```python
from build123d import *

# Parameters (mm, degrees)
SKETCH_1_R               = 5
SKETCH_1_W               = 40
SKETCH_1_H               = 6
EXTRUDE_1_DEPTH          = 2
CUT_EXTRUDE_2_DEPTH      = 46.44227107
CUT_EXTRUDE_2_DEPTH_BACK = 46.44227107
SKETCH_1_3_R             = 2
FILLET_1_R               = 3


with BuildPart() as part:
    # 草图1 → 凸台-拉伸1 (new body)
    with BuildSketch(Plane(origin=(0, 0, 0), x_dir=(0, 0, -1), z_dir=(1, 0, 0))):
        Circle(SKETCH_1_R)
        with Locations((40, -1)):
            Circle(SKETCH_1_R)
        with Locations((20, 0)):
            Rectangle(SKETCH_1_W, SKETCH_1_H)
    extrude(amount=EXTRUDE_1_DEPTH)

    # 草图1<3> → 切除-拉伸2 (cut, two sides: drawn at the far end of the back side and taken through both)
    with BuildSketch(Plane(origin=(0, 0, 0), x_dir=(0, 0, -1), z_dir=(1, 0, 0)).offset(-CUT_EXTRUDE_2_DEPTH_BACK)):
        Circle(SKETCH_1_3_R)
        with Locations((40, -1)):
            Circle(SKETCH_1_3_R)
    extrude(amount=CUT_EXTRUDE_2_DEPTH + CUT_EXTRUDE_2_DEPTH_BACK, mode=Mode.SUBTRACT)

    # 圆角1
    fillet_1_edges = [part.edges().sort_by_distance(p)[0] for p in [
        (1, -3, -35.417424305),
        (1, 3, -37),
        (1, 3, -4),
        (1, -3, -4),
    ]]
    fillet(fillet_1_edges, radius=FILLET_1_R)


solid = part.part
```
Can you work these out from the model? Positions are in its coordinate system, mm. A direction names the side the tool comes from. Coordinates: 2 decimals unless noted, no trailing zeros. Write each loop counter-clockwise with the first axis right and the second up, starting at its lowest first coordinate (ties: lowest second). Pieces come first, ordered by that corner, then holes. Notation, with made-up numbers: (47, -8) - (69, -8) arc R27 ccw to (69, 30) - close; hole circle Ø2 at (18, -34). An arc over 180 degrees is marked (long way). Return JSON: item names as keys, results as strings.
Q1. Please list where these lines run through material, in increasing order: L1, parallel to Y at x = 1.1, z = 0; L2, parallel to Z at x = 1.15, y = -1.25; L3, parallel to Z at x = 0.85, y = 0. Write a range as from..to.
Computed values:
{"L1": "y = -5..-2, 2..5", "L2": "z = -44.99..-41.98, -38.02..-1.56, 1.56..4.84", "L3": "z = -44.9..-41.73, -38.27..-2, 2..5"}
Q2. If we section it at D-D (y = 1.5): Please give me the cut outline in (x, z).
Computed values:
{"outline": "(0, -44.33) - (2, -44.33) - (2, -1.32) - (0, -1.32) - close; (0, 1.32) - (2, 1.32) - (2, 4.77) - (0, 4.77) - close"}
Q3. If we section it at A-A (z = -40): Please give me the cut outline in (x, y).
Computed values:
{"outline": "(0, -6) - (2, -6) - (2, -3) - (0, -3) - close; (0, 1) - (2, 1) - (2, 4) - (0, 4) - close"}
Q4. If we section it at B-B (y = -1): Please give me the cut outline in (x, z).
Computed values:
{"outline": "(0, -45) - (2, -45) - (2, -42) - (0, -42) - close; (0, -38) - (2, -38) - (2, -1.73) - (0, -1.73) - close; (0, 1.73) - (2, 1.73) - (2, 4.9) - (0, 4.9) - close"}
Q5. If we section it at C-C (x = 1.35): Count the separate pieces of the cut face and the enclosed holes in it, then the cut area to 3 significant figures.
Computed values:
{"separate pieces": "1", "enclosed holes": "2", "area": "317 mm2"}
Q6. I'm going to push flat-ended pins straight in: pin 1 Ø0.6 at (x, z) = (1.5, -27.5) entering from +Y; pin 2 Ø1 at (x, z) = (1, -19) entering from -Y. Where does each tip first touch, or does it pass through?
Computed values:
{"pin 1": "stops at y = 3", "pin 2": "stops at y = -3"}
Q7. On a 3-axis mill with a long thin cutter (end or side, diameter ignored), from which of +Z, -Z, +X, -X, +Y, -Y can I reach the whole of each face in a straight line? I mean faces 1 (the flat face through (2, 0, -20)), 2 (the cylindrical face through (1.01, 3.2, -4.22)), 3 (the cylindrical face through (1.014, -3.188, -4.245)). Say none if no direction works.
Computed values:
{"face 1": "+Z, -Z, +X, +Y, -Y", "face 2": "+X, -X, +Y", "face 3": "+X, -X, -Y"}
